The listing builds one solid part. Answer for the finished solid, in the listing's coordinates (mm). Coordinates: 2 decimals unless noted, no trailing zeros. Loops run counter-clockwise (first coordinate to the right, second up) from the corner with the lowest first, then second, coordinate; pieces in that order, holes last. Notation, with made-up numbers: (20.25, 48.25) - (44.25, 48.25) arc R21 ccw to (44.25, 82.25) - close; hole circle Ø3 at (-17, 69). An arc over 180 degrees is marked (long way). Put each result on its own line as item: value.
```python
from build123d import *

# Parameters (mm, degrees)
F0_W     = 31.75
F0_H     = 25.4
F1_DEPTH = 12.7
F2_R     = 4.7498
F3_DEPTH = 12.7
F4_R     = 9.525
F4_R_2   = 4.7498
F4_R_3   = 3.96875
F5_DEPTH = 3.175
F7_D     = 5.207
F4_W     = 31.75
F4_H     = 25.4
F9_DEPTH = 2.54


with BuildPart() as f1:
    # F0 (on Front) → F1 (new body)
    with BuildSketch(Plane.XZ):
        with Locations((15.875, 12.7)):
            Rectangle(F0_W, F0_H)
    extrude(amount=F1_DEPTH)

    # F2 (on face) → F3 (cut, through all)
    with BuildSketch(Plane.XZ.offset(12.7)):
        with Locations((15.875, 12.7)):
            Circle(F2_R)
    extrude(amount=-F3_DEPTH, mode=Mode.SUBTRACT)

    # F7 (through all)
    with Locations(Plane(origin=(0, 0, 0), x_dir=(1, 0, 0), z_dir=(0, 0, -1))):
        with Locations((6.35, 6.35), (25.4, 6.35)):
            Hole(F7_D / 2)

    # F4 (on face) → F9 (join)
    with BuildSketch(Plane.XZ.offset(12.7)):
        with Locations((15.875, 12.7)):
            Rectangle(F4_W, F4_H)
        with Locations((15.875, 12.7)):
            Circle(F4_R, mode=Mode.SUBTRACT)
        with Locations((15.875, 12.7)):
            Circle(F4_R)
        with Locations((15.875, 12.7)):
            Circle(F4_R_2, mode=Mode.SUBTRACT)
    extrude(amount=F9_DEPTH)


with BuildPart() as f5:
    # F4 (on face) → F5 (new body)
    with BuildSketch(Plane.XZ.offset(12.7)):
        with Locations((15.875, 12.7)):
            Circle(F4_R)
        with Locations((15.875, 12.7)):
            Circle(F4_R_2, mode=Mode.SUBTRACT)
        with Locations((15.875, 12.7)):
            Circle(F4_R_2)
        with Locations((15.875, 12.7)):
            Circle(F4_R_3, mode=Mode.SUBTRACT)
    extrude(amount=F5_DEPTH)


solid = f1.part
```
1) The part is cut by section D-D (y = -12.5). Give the vertices of the cut face in (x, z) (3 decimals), and give its area (3 significant figures).
Found:
outline: (0, 0) - (31.75, 0) - (31.75, 25.4) - (0, 25.4) - close; hole circle Ø9.5 at (15.875, 12.7)
area: 736 mm^2
2) This flat-tipped pin is pushed along its axis until it touches: pin 1 (4 mm diameter, centred on x = 25.4, y = -6.35, fed in from -Z). Where does it stop, or does it pass through?
Found:
pin 1: passes through
3) The part is cut by section A-A (z = 12.7). Give the vertices of the cut face in (x, y).
Found:
outline: (0, -15.24) - (11.13, -15.24) - (11.13, 0) - (0, 0) - close; (20.62, -15.24) - (31.75, -15.24) - (31.75, 0) - (20.62, 0) - close; hole circle Ø5.21 at (6.35, -6.35); hole circle Ø5.21 at (25.4, -6.35)
4) Straight lines are drawn through the part: L1, parallel to X at y = -6.5, z = 12.5; L2, parallel to Y at x = 25.4, z = 14; L3, parallel to Z at x = 16, y = -2.75. For each, find the intervals that lie inside material, in ascending order. Write a range as [from, to].
Found:
L1: x = [0, 3.75], [8.95, 11.13], [20.62, 22.8], [28, 31.75]
L2: y = [-15.24, -8.95], [-3.75, 0]
L3: z = [0, 7.95], [17.45, 25.4]
5) The part is cut by section C-C (x = 25.4). Give the vertices of the cut face in (y, z), and give its area (3 significant figures).
Found:
outline: (-15.24, 0) - (-8.95, 0) - (-8.95, 25.4) - (-15.24, 25.4) - close; (-3.75, 0) - (0, 0) - (0, 25.4) - (-3.75, 25.4) - close
area: 255 mm^2
6) For a pull along X with two mould halves and no side action, classify faces 1 (the face through (0, -8, 13)), 2 (the face through (3.867, -7.132, 12.878)), 3 (the face through (16, -8, 0)), 4 (the face through (31.75, -8, 13)) as pulls with the +X half, pulls with the -X half, needs draft (parallel to the pull), parting line crosses it, or undercut.
Found:
face 1: pulls with the -X half
face 2: undercut
face 3: needs draft
face 4: pulls with the +X half
7) The part is cut by section B-B (y = -4.25). Give the vertices of the cut face in (x, z) (3 decimals).
Found:
outline: (0, 0) - (4.811, 0) - (4.811, 25.4) - (0, 25.4) - close; (7.889, 0) - (23.861, 0) - (23.861, 25.4) - (7.889, 25.4) - close; (26.939, 0) - (31.75, 0) - (31.75, 25.4) - (26.939, 25.4) - close; hole circle Ø9.5 at (15.875, 12.7)
